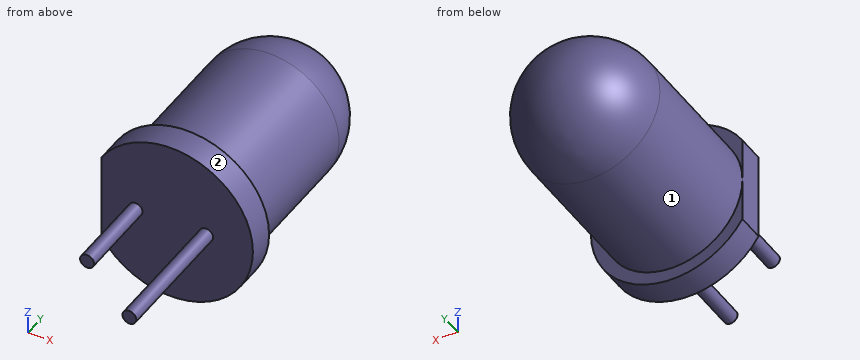
```python
from build123d import *

# Parameters (mm, degrees)
SKETCH1_R           = 2.95
BOSS_EXTRUDE1_DEPTH = 1
SKETCH2_R           = 2.5
BOSS_EXTRUDE2_DEPTH = 7.6
FILLET1_R           = 2.5
SKETCH3_R           = 0.25
BOSS_EXTRUDE3_DEPTH = 4.75
CUT_EXTRUDE1_START  = -1.75
SKETCH4_R           = 0.25
CUT_EXTRUDE1_DEPTH  = 1.75
CUT_EXTRUDE2_DEPTH  = 9.669775084


with BuildPart() as part:
    # Sketch1 → Boss-Extrude1 (new body)
    with BuildSketch(Plane(origin=(0, 0, 0), x_dir=(1, 0, 0), z_dir=(0, 1, 0))):
        with Locations(Location((0, 0, 0), (0, 0, 270))):
            Circle(SKETCH1_R)
    extrude(amount=BOSS_EXTRUDE1_DEPTH)

    # Sketch2 → Boss-Extrude2 (add)
    with BuildSketch(Plane(origin=(0, 1, 0), x_dir=(1, 0, 0), z_dir=(0, 1, 0))):
        with Locations(Location((0, 0, 0), (0, 0, 90))):
            Circle(SKETCH2_R)
    extrude(amount=BOSS_EXTRUDE2_DEPTH)

    # Fillet1
    fillet1_edges = [part.edges().sort_by_distance(p)[0] for p in [
        (0, 8.6, 2.5),
    ]]
    fillet(fillet1_edges, radius=FILLET1_R)

    # Sketch3 → Boss-Extrude3 (add)
    with BuildSketch(Plane.XZ):
        with Locations(Location((-1.27, 0, 0), (0, 0, 90))):
            Circle(SKETCH3_R)
        with Locations(Location((1.27, 0, 0), (0, 0, 90))):
            Circle(SKETCH3_R)
    extrude(amount=BOSS_EXTRUDE3_DEPTH)

    # Sketch4 → Cut-Extrude1 (cut)
    with BuildSketch(Plane.XZ.offset(4.75).offset(CUT_EXTRUDE1_START)):
        with Locations(Location((-1.27, 0, 0), (0, 0, 90))):
            Circle(SKETCH4_R)
    extrude(amount=CUT_EXTRUDE1_DEPTH, mode=Mode.SUBTRACT)

    # Sketch5 → Cut-Extrude2 (cut, through all)
    with BuildSketch(Plane(origin=(0, 1, 0), x_dir=(1, 0, 0), z_dir=(0, 1, 0))):
        Polygon((-2.5, 0), (-2.5, 1.983520803), (-3.125999015, 1.983520803), (-3.125999015, 0), (-3.125999015, -2.184477883), (-2.5, -2.184477883), align=None)
    extrude(amount=-CUT_EXTRUDE2_DEPTH, mode=Mode.SUBTRACT)


solid = part.part
```
Could you check a few things on this model? Use its own coordinates, in mm. Face numbers are marked on the shaded views. A direction names the side the tool comes from. Give positions to 0.01 mm unless a question says otherwise; leave off trailing zeros. Write each loop counter-clockwise with the first axis right and the second up, starting at its lowest first coordinate (ties: lowest second). Pieces come first, ordered by that corner, then holes. Notation, with made-up numbers: (66, -30) -> (118, -30) arc R10 cw to (118, -23) -> close; hole circle Ø4 at (-10, 43). An arc over 180 degrees is marked (long way). Write each question's results on one line, items separated by ' | '.
1. I need wall thicknesses on L1, parallel to Y at x = 0.4, z = 2.65; L2, parallel to X at y = 5, z = -0.1; L3, parallel to Z at x = 0.4, y = 5.75. Which ranges of each line are inside material? Lowest first, please.
Check sheet entries:
L1: y = 0 to 1 | L2: x = -2.5 to 2.5 | L3: z = -2.47 to 2.47
2. I want a section at A-A, the plane y = -1.25. Write out the boundary of the cut face in (x, z).
Check sheet entries:
outline: circle Ø0.5 at (-1.27, 0); circle Ø0.5 at (1.27, 0)
3. I want a section at C-C, the plane z = 2.35. Write out the boundary of the cut face in (x, y).
Check sheet entries:
outline: (-1.78, 0) -> (1.78, 0) -> (1.78, 1) -> (0.85, 1) -> (0.85, 6.1) arc R0.85 ccw to (-0.85, 6.1) -> (-0.85, 1) -> (-1.78, 1) -> close
4. I want a section at D-D, the plane y = -3.5. Write out the boundary of the cut face in (x, z).
Check sheet entries:
outline: circle Ø0.5 at (1.27, 0)
5. On a 3-axis mill with a long thin cutter (end or side, diameter ignored), from which of +Z, -Z, +X, -X, +Y, -Y can I reach the whole of each face in a straight line? I mean the marked faces 1 and 2. Say none if no direction works.
Check sheet entries:
face 1: +Y | face 2: +Y, -Y
6. I want a section at B-B, the plane x = 1.27. Write out the boundary of the cut face in (y, z), then the cut area to 3 significant figures.
Check sheet entries:
outline: (-4.75, -0.25) -> (0, -0.25) -> (0, -2.66) -> (1, -2.66) -> (1, -2.15) -> (6.1, -2.15) arc R2.15 ccw to (6.1, 2.15) -> (1, 2.15) -> (1, 2.66) -> (0, 2.66) -> (0, 0.25) -> (-4.75, 0.25) -> close | area: 36.9 mm²
7. Will these pins go through, and if not, where does the flat tip stop? pin 1 Ø0.6 at (x, z) = (-1.5, 0) entering from -Y; pin 2 Ø2 at (y, z) = (3.5, -2) entering from -X; pin 3 Ø2 at (y, z) = (-3.5, -0.5) entering from -X.
Check sheet entries:
pin 1: stops at y = -3 | pin 2: stops at x = -2.29 | pin 3: stops at x = -1.52
